from build123d import *

# Parameters (mm, degrees)
F0_W     = 2.9718
F0_H     = 6.35
F1_DEPTH = 2.9718


with BuildPart() as f1:
    # F0 (on Right) → F1 (new body)
    with BuildSketch(Plane.YZ):
        Polygon((38.1, 19.05), (38.1, 31.75), (-38.1, 31.75), (-38.1, 19.05), (-38.1, 12.7), (-38.1, -12.7), (-41.0718, -12.7), (-41.0718, -19.05), (-38.1, -19.05), (-38.1, -31.75), (-25.4, -31.75), (-25.4, -28.7782), (-20.828, -28.7782), (-20.828, -22.967306), (-23.495, -22.967306), (-23.495, -19.919306), (-20.828, -19.919306), (-20.828, -19.05), (-17.272, -19.05), (-17.272, -19.919306), (-14.605, -19.919306), (-14.605, -22.967306), (-17.272, -22.967306), (-17.272, -28.7782), (-12.7, -28.7782), (-12.7, -31.75), (12.7, -31.75), (12.7, -28.7782), (17.272, -28.7782), (17.272, -22.967306), (14.605, -22.967306), (14.605, -19.919306), (17.272, -19.919306), (17.272, -19.05), (20.828, -19.05), (20.828, -19.919306), (23.495, -19.919306), (23.495, -22.967306), (20.828, -22.967306), (20.828, -28.7782), (25.4, -28.7782), (25.4, -31.75), (38.1, -31.75), (38.1, -19.05), (41.0718, -19.05), (41.0718, -12.7), (38.1, -12.7), (38.1, 12.7), (41.0718, 12.7), (41.0718, 19.05), align=None)
        with BuildLine():
            Line((-38.1, 31.75), (38.1, 31.75))
            ThreePointArc((38.1, 31.75), (0, 69.85), (-38.1, 31.75))
        make_face()
        with Locations((-39.5859, 15.875)):
            Rectangle(F0_W, F0_H)
    extrude(amount=F1_DEPTH)


solid = f1.part
The listing builds one solid part. Answer for the finished solid, in the listing's coordinates (mm). A direction names the side the tool comes from. Give positions to 0.01 mm unless a question says otherwise; leave off trailing zeros. Write each loop counter-clockwise with the first axis right and the second up, starting at its lowest first coordinate (ties: lowest second). Pieces come first, ordered by that corner, then holes. Notation, with made-up numbers: (32.25, 74) -> (84.25, 74) arc R18 cw to (84.25, 97) -> close; hole circle Ø5 at (69, 22). An arc over 180 degrees is marked (long way). Use a Markdown table: item, result.
(1) For faces 1 (the flat face through (1, 38.1, 25)), 2 (the flat face through (1, 40, -19.05)), 3 (the flat face through (1, 22, -22.967)), 4 (the flat face through (1, -38.1, -25)), 5 (the flat face through (1, 12.7, -30)), determine the directions among +Z, -Z, +X, -X, +Y, -Y from which every point of the face is accessible in a straight line to the end or side of a thin tool.
Return value:
| item | result |
|---|---|
| face 1 | +Z, +X, -X, +Y |
| face 2 | -Z, +X, -X, +Y |
| face 3 | +X, -X |
| face 4 | -Z, +X, -X, -Y |
| face 5 | -Z, +X, -X |
(2) Flat-ended cylindrical pins translate along their axes: P1, Ø1, axis at x = 0.5, z = 42.5, coming from the -Y side; P2, Ø1.5, axis at x = 2, z = 4, coming from the -Y side; P3, Ø0.9, axis at x = 2, y = -24, coming from the -Z side. Find the tip coordinate at first contact, or state that the pin passes through.
Return value:
| item | result |
|---|---|
| P1 | y = -36.7 |
| P2 | y = -38.1 |
| P3 | z = -28.78 |
(3) Determine the mould class of faces 6 (the flat face through (1, -16, -22.967)), 7 (the flat face through (1, 0, -31.75)), 8 (the cylindrical face through (1.47, 0.84, 69.84)), 9 (the flat face through (1, -17.272, -26)) for opening direction Z: released by +Z, released by -Z, zero draft, split by the parting line, or undercut.
Return value:
| item | result |
|---|---|
| face 6 | undercut |
| face 7 | released by -Z |
| face 8 | released by +Z |
| face 9 | zero draft |
(4) Find the intervals of material crossed by probe 1 along Y at (x, z) = (0.3, -1); probe 2 along Z at (x, y) = (1, -15.5); probe 3 along Z at (x, y) = (0.4, 0), in increasing order. Write a range as from..to.
Return value:
| item | result |
|---|---|
| probe 1 | -38.1..38.1 |
| probe 2 | -28.78..-22.97, -19.92..66.55 |
| probe 3 | -31.75..69.85 |
(5) Section B-B, the plane y = -32 is taken. Determine the outline of the cut face in (x, z).
Return value:
| item | result |
|---|---|
| outline | (0, -31.75) -> (2.97, -31.75) -> (2.97, 52.43) -> (0, 52.43) -> close |
(6) Section A-A, the plane z = -2 is taken. Determine the outline of the cut face in (x, y), then the cut area to 3 significant figures.
Return value:
| item | result |
|---|---|
| outline | (0, -38.1) -> (2.97, -38.1) -> (2.97, 38.1) -> (0, 38.1) -> close |
| area | 226 mm2 |
